from build123d import *

# Parameters (mm, degrees)
F0_R     = 12.7
F1_DEPTH = 44.45
F3_DEPTH = 12.7
F4_R     = 5.08
F5_DEPTH = 63.501


with BuildPart() as f1:
    # F0 (on Front) → F1 (new body)
    with BuildSketch(Plane.XZ):
        with BuildLine():
            Line((-31.75, -8.89), (-31.75, -21.59))
            Line((-31.75, -21.59), (0, -21.59))
            Line((0, -21.59), (31.75, -21.59))
            Line((31.75, -21.59), (31.75, -8.89))
            Line((31.75, -8.89), (12.7, -8.89))
            Line((12.7, -8.89), (12.7, 0))
            Line((12.7, 0), (63.5, 0))
            Line((63.5, 0), (63.5, 12.7))
            Line((63.5, 12.7), (47.625, 12.7))
            Line((47.625, 12.7), (21.093426, 52.250173))
            ThreePointArc((21.093426, 52.250173), (0, 63.5), (-21.093426, 52.250173))
            Line((-21.093426, 52.250173), (-47.625, 12.7))
            Line((-47.625, 12.7), (-63.5, 12.7))
            Line((-63.5, 12.7), (-63.5, 0))
            Line((-63.5, 0), (-12.7, 0))
            Line((-12.7, 0), (-12.7, -8.89))
            Line((-12.7, -8.89), (-31.75, -8.89))
        make_face()
        with Locations((0, 38.1)):
            Circle(F0_R, mode=Mode.SUBTRACT)
    extrude(amount=F1_DEPTH)

    # F2 (on Front) → F3 (join)
    with BuildSketch(Plane.XZ):
        Polygon((-63.5, 63.5), (-63.5, 0), (-12.7, 0), (12.7, 0), (63.5, 0), (63.5, 63.5), align=None)
    extrude(amount=-F3_DEPTH)

    # F4 (on Top) → F5 (cut, through all)
    with BuildSketch(Plane.XY):
        with Locations((0, -22.225)):
            Circle(F4_R)
    extrude(amount=F5_DEPTH, mode=Mode.SUBTRACT)


solid = f1.part
CAD build for the part. Positions are in the model's coordinates, mm. A direction names the side the tool comes from. Give positions to 0.01 mm unless a question says otherwise; leave off trailing zeros. Write each loop counter-clockwise with the first axis right and the second up, starting at its lowest first coordinate (ties: lowest second). Pieces come first, ordered by that corner, then holes. Notation, with made-up numbers: M -34,3 L -24,3 A32 ccw -24,42 Z; hole C 76,58.25 d4. An arc over 180 degrees is marked long. Put each result on its own line as item: value. Start each with the question number.
(1) Band-saw the part on D-D, the plane z = 20. Write the cut outline in (x, y) (3 decimals).
(2) Which spindle directions (+Z, -Z, +X, -X, +Y, -Y) get a long thin tool onto all of the face, cutting with end or side? Do faces 1 (the face through (5.86, -21.914, 26.833)), 2 (the face through (-34.173, -21.914, 32.752)), 3 (the face through (45, 0, 44)). Say none if no direction does.
(3) Probe L1, parallel to Y at x = 0, z = 55.75 (3 decimals); L2, parallel to Z at x = 0, y = -16; L3, parallel to Y at x = -41.5, z = 45. List the from-to ranges inside material, lowest first.
(4) Band-saw the part on A-A, the plane x = 27. Write the cut outline in (y, z), and give its area (3 significant figures).
(5) Band-saw the part on C-C, the plane x = -49.5. Write the cut outline in (y, z), and give its area (3 significant figures).
(6) Flat gauge pins, fed straight in: pin 1 Ø2 at (x, y) = (40, 7) entering from -Z; pin 2 Ø1.5 at (y, z) = (-31, -6) entering from -X; pin 3 Ø6 at (x, y) = (-13.5, -7.5) entering from +Z. Where does each tip first touch, or does it go through?
(7) Mould opens along Y. For faces 4 (the face through (-1, 12.7, 32)), 5 (the face through (-63.5, 3, 18)), 6 (the face through (-5.075, -22.002, 56.524)) say: +Y half, -Y half, draft (parallel to the pull), parting line (faces both ways), or undercut.
(8) Band-saw the part on B-B, the plane y = -31.5. Write the cut outline in (x, z) (3 decimals), and give its area (3 significant figures).
Response values:
1. outline: M -63.5,0 L -42.728,0 L -42.728,-44.45 L 42.728,-44.45 L 42.728,0 L 63.5,0 L 63.5,12.7 L -63.5,12.7 Z; hole C 0,-22.225 d10.16
2. face 1: -Y
2. face 2: +Z, -X, -Y
2. face 3: +Z, +X, -Y
3. L1: y = -44.45 to -27.305, -17.145 to 12.7
3. L2: z = -21.59 to 25.4, 50.8 to 63.5
3. L3: y = 0 to 12.7
4. outline: M -44.45,-21.59 L 0,-21.59 L 0,-8.89 L -44.45,-8.89 Z; M -44.45,0 L 12.7,0 L 12.7,63.5 L 0,63.5 L 0,43.45 L -44.45,43.45 Z
4. area: 3,300 mm2
5. outline: M -44.45,0 L 12.7,0 L 12.7,63.5 L 0,63.5 L 0,12.7 L -44.45,12.7 Z
5. area: 1,370 mm2
6. pin 1: stops at z = 0
6. pin 2: stops at x = -12.7
6. pin 3: stops at z = 61.23
7. face 4: +Y half
7. face 5: draft
7. face 6: undercut
8. outline: M -63.5,0 L -12.7,0 L -12.7,-8.89 L -31.75,-8.89 L -31.75,-21.59 L 31.75,-21.59 L 31.75,-8.89 L 12.7,-8.89 L 12.7,0 L 63.5,0 L 63.5,12.7 L 47.625,12.7 L 21.093,52.25 A25.4 ccw -21.093,52.25 L -47.625,12.7 L -63.5,12.7 Z; hole C 0,38.1 d25.4
8. area: 5,190 mm2
